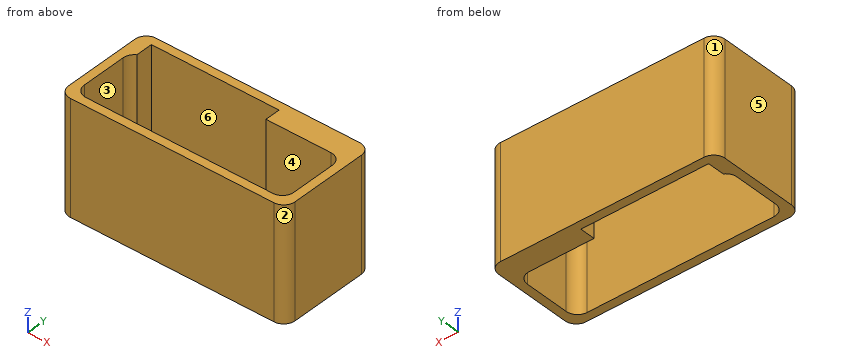
from build123d import *

# Parameters (mm, degrees)
BOSS_EXTRUDE1_DEPTH = 40


with BuildPart() as part:
    # Sketch1 → Boss-Extrude1 (new body)
    with BuildSketch(Plane.XY):
        with BuildLine():
            Line((-11.613277084, 21.495789474), (60.386722916, 21.495789474))
            ThreePointArc((60.386722916, 21.495789474), (63.21515004, 20.324216598), (64.386722916, 17.495789474))
            Line((64.386722916, 17.495789474), (64.386722916, -9.934210526))
            ThreePointArc((64.386722916, -9.934210526), (63.21515004, -12.762637651), (60.386722916, -13.934210526))
            Line((60.386722916, -13.934210526), (-11.613277084, -13.934210526))
            ThreePointArc((-11.613277084, -13.934210526), (-14.441704209, -12.762637651), (-15.613277084, -9.934210526))
            Line((-15.613277084, -9.934210526), (-15.613277084, 17.495789474))
            ThreePointArc((-15.613277084, 17.495789474), (-14.441704209, 20.324216598), (-11.613277084, 21.495789474))
        make_face()
        with BuildLine():
            Line((-10.673277084, 18.495789474), (34.456722916, 18.495789474))
            Line((34.456722916, 18.495789474), (34.456722916, 13.065789474))
            Line((34.456722916, 13.065789474), (57.386722916, 13.065789474))
            ThreePointArc((57.386722916, 13.065789474), (60.21515004, 11.894216598), (61.386722916, 9.065789474))
            Line((61.386722916, 9.065789474), (61.386722916, -6.934210526))
            ThreePointArc((61.386722916, -6.934210526), (60.21515004, -9.762637651), (57.386722916, -10.934210526))
            Line((57.386722916, -10.934210526), (-8.613277084, -10.934210526))
            ThreePointArc((-8.613277084, -10.934210526), (-11.441704209, -9.762637651), (-12.613277084, -6.934210526))
            Line((-12.613277084, -6.934210526), (-12.613277084, 9.065789474))
            ThreePointArc((-12.613277084, 9.065789474), (-12.094656121, 11.035561034), (-10.673277084, 12.494550183))
            Line((-10.673277084, 12.494550183), (-10.673277084, 13.065789474))
            Line((-10.673277084, 13.065789474), (-10.673277084, 18.495789474))
        make_face(mode=Mode.SUBTRACT)
    extrude(amount=BOSS_EXTRUDE1_DEPTH)


solid = part.part
Work out the finished part from the listing and answer in its coordinate system (mm). Face numbers are marked on the shaded views. A direction names the side the tool comes from. Round coordinates to 2 decimals unless told otherwise and drop trailing zeros. Write each loop counter-clockwise with the first axis right and the second up, starting at its lowest first coordinate (ties: lowest second). Pieces come first, ordered by that corner, then holes.
1) A cutting plane is placed at A-A (x = 47.5). Give the vertices of the cut face in (y, z), plus the area to 3 significant figures.
2) Given pin 1 Ø3 at (x, y) = (50, -9.5) entering from -Z, flat-ended and moving along its own axis, determine where the tip first touches the part or whether it passes through.
3) Straight lines are drawn through the part: line 1 (Y direction, x = 19.5, z = 19.5); line 2 (X direction, y = 3, z = 9); line 3 (Y direction, x = 53.5, z = 9.5). For each, find the intervals that lie inside material, in ascending order.
4) A cutting plane is placed at C-C (y = 16). Give the vertices of the cut face in (x, z), plus the area to 3 significant figures.
5) The mould has two halves that part along Y. Classify the marked faces 1, 2, 3 and 4: pulls with the +Y half, pulls with the -Y half, needs draft (parallel to the pull), parting line crosses it, or undercut.
6) A tool of negligible diameter and unlimited length cuts with its end or side. For the marked faces 5 and 6, from which of +Z, -Z, +X, -X, +Y, -Y can it reach the whole face along a straight path? Write none if from no direction.
7) A cutting plane is placed at B-B (z = 11). Give the vertices of the cut face in (x, y), plus the area to 3 significant figures.
Completed:
1. outline: (-13.93, 0) - (-10.93, 0) - (-10.93, 40) - (-13.93, 40) - close; (13.07, 0) - (21.5, 0) - (21.5, 40) - (13.07, 40) - close
1. area: 457 mm2
2. pin 1: stops at z = 0
3. line 1: y = -13.93 to -10.93, 18.5 to 21.5
3. line 2: x = -15.61 to -12.61, 61.39 to 64.39
3. line 3: y = -13.93 to -10.93, 13.07 to 21.5
4. outline: (-15.61, 0) - (-10.67, 0) - (-10.67, 40) - (-15.61, 40) - close; (34.46, 0) - (64.39, 0) - (64.39, 40) - (34.46, 40) - close
4. area: 1,390 mm2
5. face 1: pulls with the +Y half
5. face 2: pulls with the -Y half
5. face 3: undercut
5. face 4: undercut
6. face 5: +Z, -Z, -X, +Y, -Y
6. face 6: +Z, -Z
7. outline: (-15.61, -9.93) arc R4 ccw to (-11.61, -13.93) - (60.39, -13.93) arc R4 ccw to (64.39, -9.93) - (64.39, 17.5) arc R4 ccw to (60.39, 21.5) - (-11.61, 21.5) arc R4 ccw to (-15.61, 17.5) - close; hole (-12.61, -6.93) arc R4 ccw to (-8.61, -10.93) - (57.39, -10.93) arc R4 ccw to (61.39, -6.93) - (61.39, 9.07) arc R4 ccw to (57.39, 13.07) - (34.46, 13.07) - (34.46, 18.5) - (-10.67, 18.5) - (-10.67, 12.49) arc R4 ccw to (-12.61, 9.07) - close
7. area: 813 mm2
